Input: part model. Units: mm. Frame: model coordinates. Give positions to 0.01 mm unless a question says otherwise; leave off trailing zeros. Loops run counter-clockwise (first coordinate to the right, second up) from the corner with the lowest first, then second, coordinate; pieces in that order, holes last. Notation, with made-up numbers: (39, 23) -> (48, 23) arc R17 cw to (48, 34) -> close; hole circle Ø6 at (-26, -36). An arc over 180 degrees is marked (long way). Answer as a JSON object with one key per item and string values. Group by question number.
```python
from build123d import *

# Parameters (mm, degrees)
BOSS_EXTRUDE1_DEPTH        = 12.5
F_10_24_TAPPED_HOLE2_D     = 3.7973
F_10_24_TAPPED_HOLE2_DEPTH = 12.83
F_10_24_TAPPED_HOLE2_TIP   = 1.140824014


with BuildPart() as part:
    # Sketch1 → Boss-Extrude1 (new body, symmetric)
    with BuildSketch(Plane(origin=(0, 0, 0), x_dir=(0, 0, -1), z_dir=(1, 0, 0))):
        Polygon((0, 0), (0, 25.4), (-25.4, 10.735303163), (-25.4, 0), align=None)
    extrude(amount=BOSS_EXTRUDE1_DEPTH, both=True)

    # #10-24 Tapped Hole2
    with Locations(Plane(origin=(0, 0, 0), x_dir=(-1, 0, 0), z_dir=(0, -1, 0))):
        with Locations((105.780967711, 37.577069838), (0, -12.7)):
            Hole(F_10_24_TAPPED_HOLE2_D / 2, depth=F_10_24_TAPPED_HOLE2_DEPTH)
            with Locations((0, 0, -(F_10_24_TAPPED_HOLE2_DEPTH + F_10_24_TAPPED_HOLE2_TIP / 2))):  # 118° drill point
                Cone(0, F_10_24_TAPPED_HOLE2_D / 2, F_10_24_TAPPED_HOLE2_TIP, mode=Mode.SUBTRACT)


solid = part.part
```
Q1. Pull-direction query (Z, two-part tool) for faces 1 (the face through (0, 13, 0)), 2 (the face through (-0.247, 6.505, 10.818)), 3 (the face through (0, 5, 25.4)); classes: +Z half, -Z half, draft (parallel to the pull), parting line (faces both ways), or undercut.
Q2. Section C-C on y = 15.25. Return the cut outline in (x, z), then the cut area to 3 significant figures.
Q3. Section A-A on y = 5.25. Return the cut outline in (x, z).
Q4. Pin query (flat end, axial travel): pin 1 Ø8 at (x, z) = (8.5, 6) entering from +Y; pin 2 Ø10 at (x, z) = (2.5, 7.5) entering from +Y; pin 3 Ø1.5 at (x, y) = (7, 18) entering from +Z. Return the tip coordinate at first contact, or that it passes through.
Q5. Section B-B on x = 10. Return the cut outline in (y, z).
Q6. Ray query, probe 1 along Z at (x, y) = (0, 9.5); probe 2 along X at (y, z) = (10.25, 12.7); probe 3 along Z at (x, y) = (-4, 20.5). Return the intervals inside material, ascending.
Numbers:
{
 "1": {"face 1": "-Z half", "face 2": "undercut", "face 3": "+Z half"},
 "2": {"outline": "(-12.5, 0) -> (12.5, 0) -> (12.5, 17.58) -> (-12.5, 17.58) -> close", "area": "440 mm²"},
 "3": {"outline": "(-12.5, 0) -> (12.5, 0) -> (12.5, 25.4) -> (-12.5, 25.4) -> close; hole circle Ø3.8 at (0, 12.7)"},
 "4": {"pin 1": "stops at y = 24.25", "pin 2": "stops at y = 23.96", "pin 3": "stops at z = 14.12"},
 "5": {"outline": "(0, 0) -> (25.4, 0) -> (10.74, 25.4) -> (0, 25.4) -> close"},
 "6": {"probe 1": "z = 0 to 10.8, 14.6 to 25.4", "probe 2": "x = -12.5 to -1.9, 1.9 to 12.5", "probe 3": "z = 0 to 8.49"}
}
